Design review of the part built by this model. Coordinates are the model's own, in mm. A direction names the side the tool comes from. Coordinates: 2 decimals unless noted, no trailing zeros. Order: outer loops, then holes, each group sorted by start corner. A loop starts at its lowest first (then second) coordinate and runs counter-clockwise, first axis right, second up. Notation, with made-up numbers: (58, 75) -> (92, 75) arc R24 cw to (92, 113) -> close; hole circle Ø11 at (29, 67.25). An arc over 180 degrees is marked (long way). Use a Markdown table: item, result. Add a question column.
Q1. Add section A-A (y = -11.5). State the section outline as (x, z) points (3 decimals).
Q2. Wall thickness on probe 1 along Y at (x, z) = (0, 18); probe 2 along Y at (x, z) = (0, 20.2); probe 3 along Z at (x, y) = (11.5, 8): over which ranges is each line inside the solid? List them lowest first.
Q3. Add section B-B (x = -3.5). State the section outline as (y, z) points.
Q4. Add section D-D (y = 0). State the section outline as (x, z) points (3 decimals), then the cut area to 3 significant figures.
Q5. Machinability: for faces 4 (the face through (-12, 5, -24.161)), 5 (the face through (10, 5, -26)), 6 (the face through (0, -2, 19.161)), 7 (the face through (2, 0, 16.161)), which of the approach directions +Z, -Z, +X, -X, +Y, -Y give a long, thin tool a straight path to every point of the face, cutting with its end or side? Answer none if there is none.
Q6. Insertion check: pin 1 (1.5 mm diameter, centred on x = -7, z = 15, fed in from +Y); pin 2 (3.5 mm diameter, centred on x = 0, y = 15, fed in from -Z); pin 3 (3.5 mm diameter, centred on y = 6.5, z = -26, fed in from +X); pin 4 (2.5 mm diameter, centred on x = 0, y = 0, fed in from +Z). Each pin has a flat end and moves straight along its axis. Give the tip position at first contact, or say it passes through.
Q7. Add section C-C (z = -15). State the section outline as (x, y) points, then the cut area to 3 significant figures.
Q8. The part is to be moulded in two halves that separate along X. For faces 1 (the face through (-0.54, -17.44, 20.18)), 2 (the face through (-28.436, 0.42, -3.404)), 3 (the face through (-4, 0, 21.161)), say which applies: pulls with the +X half, pulls with the -X half, needs draft (parallel to the pull), parting line crosses it, or undercut.
from build123d import *

# Parameters (mm, degrees)
BOSS_EXTRUDE1_DEPTH = 30
CUT_EXTRUDE1_DEPTH  = 50
SKETCH5_R           = 1.5
CUT_EXTRUDE2_DEPTH  = 5
SKETCH5_3_R         = 2.5
SKETCH5_3_R_2       = 1.5
CUT_EXTRUDE3_DEPTH  = 2
LPATTERN1_COUNT     = 2
LPATTERN1_PITCH     = 15
LPATTERN1_COL_COUNT = 2
LPATTERN1_COL_PITCH = 15


with BuildPart() as part:
    # Sketch1 → Boss-Extrude1 (new body, symmetric)
    with BuildSketch(Plane(origin=(0, 0, 0), x_dir=(1, 0, 0), z_dir=(0, 1, 0))):
        with BuildLine():
            Line((-15, -21.161374477), (15, -21.161374477))
            ThreePointArc((15, -21.161374477), (28.43891729, 3), (15, 27.161374477))
            Line((15, 27.161374477), (-15, 27.161374477))
            ThreePointArc((-15, 27.161374477), (-28.43891729, 3), (-15, -21.161374477))
        make_face()
        with BuildLine():
            Line((-10, -16.161374477), (10, -16.161374477))
            ThreePointArc((10, -16.161374477), (0, 19.005), (-10, -16.161374477))
        make_face(mode=Mode.SUBTRACT)
    extrude(amount=BOSS_EXTRUDE1_DEPTH, both=True)

    # Sketch4 → Cut-Extrude1 (cut)
    with BuildSketch(Plane(origin=(0, 30, 0), x_dir=(1, 0, 0), z_dir=(0, 1, 0))):
        Polygon((-10, 27.161374477), (-10, 24.161374477), (-13.5, 24.161374477), (-13.5, 20.661374477), (13.5, 20.661374477), (13.5, 24.161374477), (10, 24.161374477), (10, 27.161374477), align=None)
    extrude(amount=-CUT_EXTRUDE1_DEPTH, mode=Mode.SUBTRACT)

    # Sketch5 → Cut-Extrude2 (cut)
    with BuildSketch(Plane.XY.offset(21.161374477)):
        Circle(SKETCH5_R)
    cut_extrude2 = extrude(amount=-CUT_EXTRUDE2_DEPTH, mode=Mode.SUBTRACT)

    # Sketch5<3> → Cut-Extrude3 (cut)
    with BuildSketch(Plane.XY.offset(21.161374477)):
        Circle(SKETCH5_3_R)
        Circle(SKETCH5_3_R_2, mode=Mode.SUBTRACT)
    cut_extrude3 = extrude(amount=-CUT_EXTRUDE3_DEPTH, mode=Mode.SUBTRACT)

    # LPattern1: Cut-Extrude2, Cut-Extrude3 ×2
    with Locations(*[(0, -i * LPATTERN1_PITCH, 0) for i in range(1, LPATTERN1_COUNT)]):
        add(cut_extrude2, mode=Mode.SUBTRACT)
        add(cut_extrude3, mode=Mode.SUBTRACT)

    # LPattern1 col: Cut-Extrude2, Cut-Extrude3 ×2
    with Locations(*[(0, i * LPATTERN1_COL_PITCH, 0) for i in range(1, LPATTERN1_COL_COUNT)]):
        add(cut_extrude2, mode=Mode.SUBTRACT)
        add(cut_extrude3, mode=Mode.SUBTRACT)


solid = part.part
Established:
| question | item | result |
|---|---|---|
| 1 | outline | (-15, -27.161) -> (-10, -27.161) -> (-10, -24.161) -> (-13.5, -24.161) -> (-13.5, -20.661) -> (13.5, -20.661) -> (13.5, -24.161) -> (10, -24.161) -> (10, -27.161) -> (15, -27.161) arc R28.439 ccw to (15, 21.161) -> (-15, 21.161) arc R28.439 ccw to start; hole (-10, 16.161) arc R19.005 ccw (long way) to (10, 16.161) -> close |
| 2 | probe 1 | -30 to -16.5, -13.5 to -1.5, 1.5 to 13.5, 16.5 to 30 |
| 2 | probe 2 | -30 to -17.5, -12.5 to -2.5, 2.5 to 12.5, 17.5 to 30 |
| 2 | probe 3 | -27.16 to -24.16, -20.66 to -15.13, 15.13 to 21.16 |
| 3 | outline | (-30, -27.16) -> (-20, -27.16) -> (-20, -20.66) -> (30, -20.66) -> (30, -18.68) -> (-30, -18.68) -> close; (-30, 16.16) -> (30, 16.16) -> (30, 21.16) -> (-30, 21.16) -> close |
| 4 | outline | (-15, -27.161) -> (-10, -27.161) -> (-10, -24.161) -> (-13.5, -24.161) -> (-13.5, -20.661) -> (13.5, -20.661) -> (13.5, -24.161) -> (10, -24.161) -> (10, -27.161) -> (15, -27.161) arc R28.439 ccw to (15, 21.161) -> (2.5, 21.161) -> (2.5, 19.161) -> (1.5, 19.161) -> (1.5, 16.161) -> (10, 16.161) arc R19.005 cw (long way) to (-10, 16.161) -> (-1.5, 16.161) -> (-1.5, 19.161) -> (-2.5, 19.161) -> (-2.5, 21.161) -> (-15, 21.161) arc R28.439 ccw to start |
| 4 | area | 1,100 mm^2 |
| 5 | face 4 | +Y |
| 5 | face 5 | -Z, +Y |
| 5 | face 6 | +Z |
| 5 | face 7 | +Y, -Y |
| 6 | pin 1 | through |
| 6 | pin 2 | z = -20.66 |
| 6 | pin 3 | x = 18.9 |
| 6 | pin 4 | z = -18.96 |
| 7 | outline | (-25.78, -30) -> (-11.67, -30) -> (-11.67, 30) -> (-25.78, 30) -> close; (11.67, -30) -> (25.78, -30) -> (25.78, 30) -> (11.67, 30) -> close |
| 7 | area | 1,690 mm^2 |
| 8 | face 1 | undercut |
| 8 | face 2 | pulls with the -X half |
| 8 | face 3 | needs draft |
